Autodesk Inventor part; units mm, degrees
ref_plane "YZ Plane" through (0, 0, 0) normal (1, 0, 0) x (0, 1, 0)
ref_plane "XZ Plane" through (0, 0, 0) normal (0, 1, 0) x (-1, 0, 0)
ref_plane "XY Plane" through (0, 0, 0) normal (0, 0, 1) x (1, 0, 0)
sketch "Sketch2" plane through (0, 0, 0) normal (0, 0, 1) x (1, 0, 0)
  circle A0 centre (4.0931, -20.1479) radius 2.1844 construction
  line L0 (57.7016, -119.5892) -> (56.531, -118.5169) construction
  circle A1 centre (58.0948, -128.5608) radius 2.1844 construction
  arc A2 (56.1046, -127.9465) -> (60.1543, -128.2505) centre (58.0948, -128.5608) ccw
  arc A3 (5.9348, -19.175) -> (2.2886, -21.1879) centre (4.0931, -20.1479) ccw
  arc A4 (54.75, -127.2766) -> (61.6095, -127.8658) centre (58.0948, -128.5608) ccw
  arc A5 (7.2676, -18.4867) -> (0.9949, -21.9473) centre (4.0931, -20.1479) ccw
  line L1 (54.75, -127.2766) -> (57.7016, -119.5892)
  line L2 (57.7016, -119.5892) -> (0.9949, -21.9473)
  line L3 (2.2886, -21.1879) -> (58.7941, -119.2338)
  line L4 (58.7941, -119.2338) -> (56.1046, -127.9465)
  line L5 (60.1543, -128.2505) -> (58.7957, -119.2343)
  line L6 (58.7957, -119.2343) -> (5.9348, -19.175)
  line L7 (7.2676, -18.4867) -> (59.8498, -118.9661)
  line L8 (59.8498, -118.9661) -> (61.6095, -127.8658)
  point P0 (0, 0)
  dimension "d17" = 4.1656
  dimension "d18" = 4.1656
  dimension "d19" = 1.5
  dimension "d20" = 1.5
  dimension "d21" = 1
extrude "Extrusion2" add sketch "Sketch2" along normal blind 5
properties part number "Angle Changer left band"
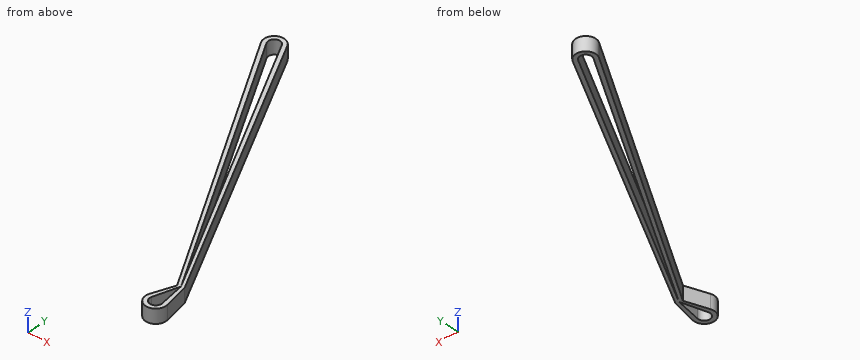
CAD build for the part. Positions are in the model's coordinates, mm. Round coordinates to 2 decimals unless told otherwise and drop trailing zeros. Write each loop counter-clockwise with the first axis right and the second up, starting at its lowest first coordinate (ties: lowest second). Pieces come first, ordered by that corner, then holes.
Item 1: Band-saw the part on C-C on y = -43.5. Write the cut outline in (x, z).
Filled in:
outline: (13.51, 0) - (15.15, 0) - (15.15, 5) - (13.51, 5) - close; (18.79, 0) - (20.36, 0) - (20.36, 5) - (18.79, 5) - close
Item 2: Drop flat-ended pins along their axis: pin 1 Ø1 at (y, z) = (-103, 3) entering from +X; pin 2 Ø3 at (x, z) = (44.5, 4) entering from -Y. Give the stop position or say it passes through.
Filled in:
pin 1: stops at x = 51.76
pin 2: stops at y = -99.44
Item 3: Drill centre lines: L1, parallel to X at y = -48.5, z = 1.15; L2, parallel to X at y = -59, z = 3.5; L3, parallel to Y at x = 24, z = 2.8. Where is each one in solid material? Low to high.
Filled in:
L1: x = 16.42 to 18.03, 21.43 to 22.97
L2: x = 22.51 to 24.08, 26.97 to 28.47
L3: y = -61.56 to -58.86, -53.37 to -50.46
Item 4: Band-saw the part on B-B on x = 29.5. Write the cut outline in (y, z), then the cut area to 3 significant figures.
Filled in:
outline: (-71.03, 0) - (-68.4, 0) - (-68.4, 5) - (-71.03, 5) - close; (-63.78, 0) - (-60.97, 0) - (-60.97, 5) - (-63.78, 5) - close
area: 27.2 mm2
